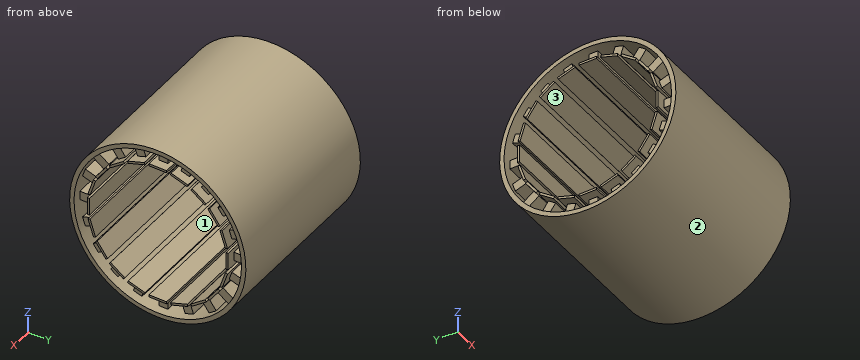
from build123d import *

# Parameters (mm, degrees)
SKETCH2_R           = 50.8
SKETCH2_R_2         = 48.26
BOSS_EXTRUDE1_DEPTH = 50.8
SKETCH3_W           = 5.08
SKETCH3_H           = 7.62
BOSS_EXTRUDE2_DEPTH = 45.72
SKETCH4_W           = 101.6
SKETCH4_H           = 10.16
BOSS_EXTRUDE3_DEPTH = 1.27
CIRPATTERN1_COUNT   = 20


with BuildPart() as part:
    # Sketch2 → Boss-Extrude1 (new body, symmetric)
    with BuildSketch(Plane(origin=(0, 0, 0), x_dir=(0, 0, -1), z_dir=(1, 0, 0))):
        Circle(SKETCH2_R)
        Circle(SKETCH2_R_2, mode=Mode.SUBTRACT)
    extrude(amount=BOSS_EXTRUDE1_DEPTH, both=True)

    # Sketch3 → Boss-Extrude2 (add, symmetric)
    with BuildSketch(Plane(origin=(0, 0, 0), x_dir=(0, 0, -1), z_dir=(1, 0, 0))):
        with Locations((0, -44.45)):
            Rectangle(SKETCH3_W, SKETCH3_H)
    boss_extrude2 = extrude(amount=BOSS_EXTRUDE2_DEPTH, both=True)

    # Sketch4 → Boss-Extrude3 (add)
    with BuildSketch(Plane(origin=(0, -40.64, 0), x_dir=(1, 0, 0), z_dir=(0, 1, 0))):
        Rectangle(SKETCH4_W, SKETCH4_H)
    boss_extrude3 = extrude(amount=BOSS_EXTRUDE3_DEPTH)

    # CirPattern1: Boss-Extrude2, Boss-Extrude3 ×20 about axis
    cirpattern1_axis = Axis((0, 0, 0), (1, 0, 0))
    for i in range(1, CIRPATTERN1_COUNT):
        add(boss_extrude2.rotate(cirpattern1_axis, i * 360 / CIRPATTERN1_COUNT))
        add(boss_extrude3.rotate(cirpattern1_axis, i * 360 / CIRPATTERN1_COUNT))


solid = part.part
CAD build for the part. Positions are in the model's coordinates, mm. Face numbers are marked on the shaded views. Round coordinates to 2 decimals unless told otherwise and drop trailing zeros. Loops run counter-clockwise (first coordinate to the right, second up) from the corner with the lowest first, then second, coordinate; pieces in that order, holes last.
(1) Cut at D-D (y = 24). Give the cut face in (x, z), plus the area to 3 significant figures.
(2) Cut at A-A (y = 0). Give the cut face in (x, z).
(3) Drop flat-ended pins along their axis: pin 1 (2 mm diameter, centred on y = -29.5, z = -21.5, fed in from +X); pin 2 (7 mm diameter, centred on y = 27, z = -35.5, fed in from -X); pin 3 (5 mm diameter, centred on x = 33.5, z = -26.5, fed in from -Y); pin 4 (1 mm diameter, centred on x = 29.5, y = -1.5, fed in from +Z). Give the stop position or say it passes through.
(4) Two-plate mould, pull along Z, no slides. Class the marked faces 1, 2 and 3: +Z half, -Z half, draft (parallel to the pull), parting line (faces both ways), or undercut.
(5) Wall check: line 1 along Y through (x, z) = (0, 0); line 2 along Y through (x, z) = (-10.5, 32). Give the ranges that are in metal, low to high.
(6) Cut at C-C (z = -23.5). Give the cut face in (x, y), plus the area to 3 significant figures.
Findings below:
1. outline: (-50.8, -44.77) - (50.8, -44.77) - (50.8, -41.87) - (-50.8, -41.87) - close; (-50.8, -32.8) - (-45.72, -32.8) - (-45.72, -37.35) - (45.72, -37.35) - (45.72, -32.8) - (50.8, -32.8) - (50.8, -31.23) - (-50.8, -31.23) - close; (-50.8, 31.23) - (50.8, 31.23) - (50.8, 32.8) - (45.72, 32.8) - (45.72, 37.35) - (-45.72, 37.35) - (-45.72, 32.8) - (-50.8, 32.8) - close; (-50.8, 41.87) - (50.8, 41.87) - (50.8, 44.77) - (-50.8, 44.77) - close
1. area: 1,740 mm2
2. outline: (-50.8, -50.8) - (50.8, -50.8) - (50.8, -48.26) - (45.72, -48.26) - (45.72, -40.64) - (50.8, -40.64) - (50.8, -39.37) - (-50.8, -39.37) - (-50.8, -40.64) - (-45.72, -40.64) - (-45.72, -48.26) - (-50.8, -48.26) - close; (-50.8, 39.37) - (50.8, 39.37) - (50.8, 40.64) - (45.72, 40.64) - (45.72, 48.26) - (50.8, 48.26) - (50.8, 50.8) - (-50.8, 50.8) - (-50.8, 48.26) - (-45.72, 48.26) - (-45.72, 40.64) - (-50.8, 40.64) - close
3. pin 1: passes through
3. pin 2: stops at x = -45.72
3. pin 3: stops at y = -44.77
3. pin 4: stops at z = 50.79
4. face 1: undercut
4. face 2: parting line
4. face 3: undercut
5. line 1: y = -50.8 to -39.37, 39.37 to 50.8
5. line 2: y = -39.45 to -36.13, -26.39 to -22.94, 22.94 to 26.39, 36.13 to 39.45
6. outline: (-50.8, -45.04) - (50.8, -45.04) - (50.8, -42.15) - (-50.8, -42.15) - close; (-50.8, -33.16) - (-45.72, -33.16) - (-45.72, -36.67) - (45.72, -36.67) - (45.72, -33.16) - (50.8, -33.16) - (50.8, -31.59) - (-50.8, -31.59) - close; (-50.8, 31.59) - (50.8, 31.59) - (50.8, 33.16) - (45.72, 33.16) - (45.72, 36.67) - (-45.72, 36.67) - (-45.72, 33.16) - (-50.8, 33.16) - close; (-50.8, 42.15) - (50.8, 42.15) - (50.8, 45.04) - (-50.8, 45.04) - close
6. area: 1,550 mm2
